Geometry: final body of the model. Coordinates: model frame, mm. Face numbers are marked on the shaded views. A direction names the side the tool comes from. Round coordinates to 2 decimals unless told otherwise and drop trailing zeros. Order: outer loops, then holes, each group sorted by start corner. A loop starts at its lowest first (then second) coordinate and runs counter-clockwise, first axis right, second up. Notation, with made-up numbers: (36, -30.75) -> (90, -30.75) arc R28 ccw to (90, -7.75) -> close; hole circle Ø1 at (37.25, 70). An arc over 180 degrees is marked (long way). Put each result on its own line as item: value.
```python
from build123d import *

# Parameters (mm, degrees)
SKETCH1_W                 = 44
SKETCH1_H                 = 57
BOSS_EXTRUDE1_DEPTH       = 2
BOSS_EXTRUDE2_DEPTH       = 3.5
BOSS_EXTRUDE2_DEPTH_BACK  = 2
SKETCH17_W                = 47.024890074
SKETCH17_H                = 2
BOSS_EXTRUDE7_DEPTH       = 38
SKETCH8_W                 = 31.89
SKETCH8_H                 = 7.76
BOSS_EXTRUDE5_DEPTH       = 9.38
SKETCH9_R                 = 2.4
CUT_EXTRUDE1_DEPTH        = 9.38
SKETCH10_R                = 3.1
CUT_EXTRUDE2_DEPTH        = 0.8
SKETCH11_R                = 3.1
CUT_EXTRUDE3_DEPTH        = 0.8
SKETCH14_R                = 2.4
CUT_EXTRUDE5_DEPTH        = 77.6
SKETCH15_R                = 3.1
CUT_EXTRUDE6_DEPTH        = 0.8
SKETCH16_R                = 3.1
CUT_EXTRUDE7_DEPTH        = 0.8
FILLET1_R                 = 1.3
FILLET2_R                 = 1.3
FILLET3_R                 = 1.3
FILLET4_R                 = 1.3
FILLET5_R                 = 1.3
FILLET7_R                 = 4
FILLET8_R                 = 4
FILLET9_R                 = 4
FILLET10_R                = 4
SKETCH19_W                = 3
SKETCH19_H                = 47
BOSS_EXTRUDE9_DEPTH       = 3.5
SKETCH20_W                = 25
SKETCH20_H                = 40
CUT_EXTRUDE8_DEPTH        = 10.38
SKETCH21_W                = 35
SKETCH21_H                = 50
CUT_EXTRUDE9_DEPTH        = 3.5
BOSS_EXTRUDE10_DEPTH      = 2.5
BOSS_EXTRUDE10_DEPTH_BACK = 2
FILLET11_R                = 2.5
FILLET12_R                = 2.5


with BuildPart() as part:
    # Sketch1 → Boss-Extrude1 (new body)
    with BuildSketch(Plane(origin=(0, 0, 0), x_dir=(1, 0, 0), z_dir=(0, 1, 0))):
        with Locations((22, 28.5)):
            Rectangle(SKETCH1_W, SKETCH1_H)
    extrude(amount=BOSS_EXTRUDE1_DEPTH)

    # Sketch2 → Boss-Extrude2 (add, two sides)
    with BuildSketch(Plane(origin=(0, 2, 0), x_dir=(1, 0, 0), z_dir=(0, 1, 0))) as boss_extrude2_sk:
        Polygon((0, 0), (0, 5), (-3, 5), (-3, 0), (-3, -3), (5, -3), (5, 0), align=None)
        Polygon((47, 0), (47, -3), (39, -3), (39, 0), (44, 0), (44, 5), (47, 5), align=None)
        Polygon((47, 57), (47, 52), (44, 52), (44, 57), (39, 57), (39, 60), (47, 60), align=None)
        Polygon((-3, 57), (-3, 60), (5, 60), (5, 57), (0, 57), (0, 52), (-3, 52), align=None)
    extrude(amount=BOSS_EXTRUDE2_DEPTH)
    extrude(boss_extrude2_sk.sketch, amount=-BOSS_EXTRUDE2_DEPTH_BACK)

    # Sketch17 → Boss-Extrude7 (add)
    with BuildSketch(Plane.ZY):
        with Locations((-28.487554963, 1)):
            Rectangle(SKETCH17_W, SKETCH17_H)
    extrude(amount=BOSS_EXTRUDE7_DEPTH)

    # Sketch8 → Boss-Extrude5 (add)
    with BuildSketch(Plane(origin=(0, 2, 0), x_dir=(1, 0, 0), z_dir=(0, 1, 0))):
        with Locations((22.150732417, 60.88)):
            Rectangle(SKETCH8_W, SKETCH8_H)
        with Locations((22.150732417, -3.88)):
            Rectangle(SKETCH8_W, SKETCH8_H)
    extrude(amount=-BOSS_EXTRUDE5_DEPTH)

    # Sketch9 → Cut-Extrude1 (cut)
    with BuildSketch(Plane(origin=(0, 0, -64.76), x_dir=(-1, 0, 0), z_dir=(0, 0, -1))):
        with Locations((-33.633843379, -3.383703118)):
            Circle(SKETCH9_R)
        with Locations((-25.663843379, -3.383703118)):
            Circle(SKETCH9_R)
        with Locations((-17.693843379, -3.383703118)):
            Circle(SKETCH9_R)
        with Locations((-9.723843379, -3.383703118)):
            Circle(SKETCH9_R)
    extrude(amount=-CUT_EXTRUDE1_DEPTH, mode=Mode.SUBTRACT)

    # Sketch10 → Cut-Extrude2 (cut)
    with BuildSketch(Plane(origin=(0, 0, -64.76), x_dir=(-1, 0, 0), z_dir=(0, 0, -1))):
        with Locations((-33.633843379, -3.383703118)):
            Circle(SKETCH10_R)
        with Locations((-25.663843379, -3.383703118)):
            Circle(SKETCH10_R)
        with Locations((-17.693843379, -3.383703118)):
            Circle(SKETCH10_R)
        with Locations((-9.723843379, -3.383703118)):
            Circle(SKETCH10_R)
    extrude(amount=-CUT_EXTRUDE2_DEPTH, mode=Mode.SUBTRACT)

    # Sketch11 → Cut-Extrude3 (cut)
    with BuildSketch(Plane.XY.offset(-57)):
        with Locations((33.633843379, -3.383703118)):
            Circle(SKETCH11_R)
        with Locations((25.633843379, -3.383703118)):
            Circle(SKETCH11_R)
        with Locations((17.633843379, -3.383703118)):
            Circle(SKETCH11_R)
        with Locations((9.633843379, -3.383703118)):
            Circle(SKETCH11_R)
    extrude(amount=-CUT_EXTRUDE3_DEPTH, mode=Mode.SUBTRACT)

    # Sketch14 → Cut-Extrude5 (cut)
    with BuildSketch(Plane.XY.offset(7.76)):
        with Locations((9.723843379, -3.383703118)):
            Circle(SKETCH14_R)
        with Locations((17.693843379, -3.383703118)):
            Circle(SKETCH14_R)
        with Locations((25.663843379, -3.383703118)):
            Circle(SKETCH14_R)
        with Locations((33.633843379, -3.383703118)):
            Circle(SKETCH14_R)
    extrude(amount=-CUT_EXTRUDE5_DEPTH, mode=Mode.SUBTRACT)

    # Sketch15 → Cut-Extrude6 (cut)
    with BuildSketch(Plane.XY.offset(7.76)):
        with Locations((9.723843379, -3.383703118)):
            Circle(SKETCH15_R)
        with Locations((17.693843379, -3.383703118)):
            Circle(SKETCH15_R)
        with Locations((25.663843379, -3.383703118)):
            Circle(SKETCH15_R)
        with Locations((33.633843379, -3.383703118)):
            Circle(SKETCH15_R)
    extrude(amount=-CUT_EXTRUDE6_DEPTH, mode=Mode.SUBTRACT)

    # Sketch16 → Cut-Extrude7 (cut)
    with BuildSketch(Plane(origin=(0, 0, 0), x_dir=(-1, 0, 0), z_dir=(0, 0, -1))):
        with Locations((-9.723843379, -3.383703118)):
            Circle(SKETCH16_R)
        with Locations((-17.693843379, -3.383703118)):
            Circle(SKETCH16_R)
        with Locations((-25.663843379, -3.383703118)):
            Circle(SKETCH16_R)
        with Locations((-33.633843379, -3.383703118)):
            Circle(SKETCH16_R)
    extrude(amount=-CUT_EXTRUDE7_DEPTH, mode=Mode.SUBTRACT)

    # Fillet1
    fillet1_edges = [part.edges().sort_by_distance(p)[0] for p in [
        (47, 5.5, -56),
        (43, 5.5, -60),
    ]]
    fillet(fillet1_edges, radius=FILLET1_R)

    # Fillet2
    fillet2_edges = [part.edges().sort_by_distance(p)[0] for p in [
        (47, 5.5, -1),
        (43, 5.5, 3),
    ]]
    fillet(fillet2_edges, radius=FILLET2_R)

    # Fillet3
    fillet3_edges = [part.edges().sort_by_distance(p)[0] for p in [
        (-3, 5.5, -56),
        (1, 5.5, -60),
    ]]
    fillet(fillet3_edges, radius=FILLET3_R)

    # Fillet4
    fillet4_edges = [part.edges().sort_by_distance(p)[0] for p in [
        (-3, 5.5, -1),
        (1, 5.5, 3),
    ]]
    fillet(fillet4_edges, radius=FILLET4_R)

    # Fillet5
    fillet5_edges = [part.edges().sort_by_distance(p)[0] for p in [
        (22.150732417, 2, -64.76),
    ]]
    fillet(fillet5_edges, radius=FILLET5_R)

    # Fillet7
    fillet7_edges = [part.edges().sort_by_distance(p)[0] for p in [
        (6.205732417, -7.38, -60.88),
    ]]
    fillet(fillet7_edges, radius=FILLET7_R)

    # Fillet8
    fillet8_edges = [part.edges().sort_by_distance(p)[0] for p in [
        (38.095732417, -7.38, -60.88),
    ]]
    fillet(fillet8_edges, radius=FILLET8_R)

    # Fillet9
    fillet9_edges = [part.edges().sort_by_distance(p)[0] for p in [
        (38.095732417, -7.38, 3.88),
    ]]
    fillet(fillet9_edges, radius=FILLET9_R)

    # Fillet10
    fillet10_edges = [part.edges().sort_by_distance(p)[0] for p in [
        (6.205732417, -7.38, 3.88),
    ]]
    fillet(fillet10_edges, radius=FILLET10_R)

    # Sketch19 → Boss-Extrude9 (add)
    with BuildSketch(Plane(origin=(0, 2, 0), x_dir=(1, 0, 0), z_dir=(0, 1, 0))):
        with Locations((-1.5, 28.5)):
            Rectangle(SKETCH19_W, SKETCH19_H)
    extrude(amount=BOSS_EXTRUDE9_DEPTH)

    # Sketch20 → Cut-Extrude8 (cut, through all)
    with BuildSketch(Plane(origin=(0, 2, 0), x_dir=(1, 0, 0), z_dir=(0, 1, 0))):
        with Locations((-20.5, 28.5)):
            Rectangle(SKETCH20_W, SKETCH20_H)
    extrude(amount=-CUT_EXTRUDE8_DEPTH, mode=Mode.SUBTRACT)

    # Sketch21 → Cut-Extrude9 (cut)
    with BuildSketch(Plane(origin=(0, 2, 0), x_dir=(1, 0, 0), z_dir=(0, 1, 0))):
        with Locations((22, 28.25)):
            Rectangle(SKETCH21_W, SKETCH21_H)
    extrude(amount=-CUT_EXTRUDE9_DEPTH, mode=Mode.SUBTRACT)

    # Sketch22 → Boss-Extrude10 (add, two sides)
    with BuildSketch(Plane(origin=(0, 2, 0), x_dir=(1, 0, 0), z_dir=(0, 1, 0))) as boss_extrude10_sk:
        Polygon((-38, 52), (-32.9998846, 52), (-32.9998846, 55.005068645), (-38, 55.005068645), (-40.988316888, 55.005068645), (-40.988316888, 46.981993776), (-38, 46.981993776), align=None)
        Polygon((-32.9998846, 4.975109926), (-32.9998846, 1.970041281), (-38, 1.970041281), (-40.988316888, 1.970041281), (-40.988316888, 9.99311615), (-38, 9.99311615), (-38, 4.975109926), align=None)
    extrude(amount=BOSS_EXTRUDE10_DEPTH)
    extrude(boss_extrude10_sk.sketch, amount=-BOSS_EXTRUDE10_DEPTH_BACK)

    # Fillet11
    fillet11_edges = [part.edges().sort_by_distance(p)[0] for p in [
        (-36.994100744, 4.5, -55.005068645),
        (-40.988316888, 4.5, -50.99353121),
    ]]
    fillet(fillet11_edges, radius=FILLET11_R)

    # Fillet12
    fillet12_edges = [part.edges().sort_by_distance(p)[0] for p in [
        (-40.988316888, 4.5, -5.981578716),
        (-36.994100744, 4.5, -1.970041281),
    ]]
    fillet(fillet12_edges, radius=FILLET12_R)


solid = part.part
```
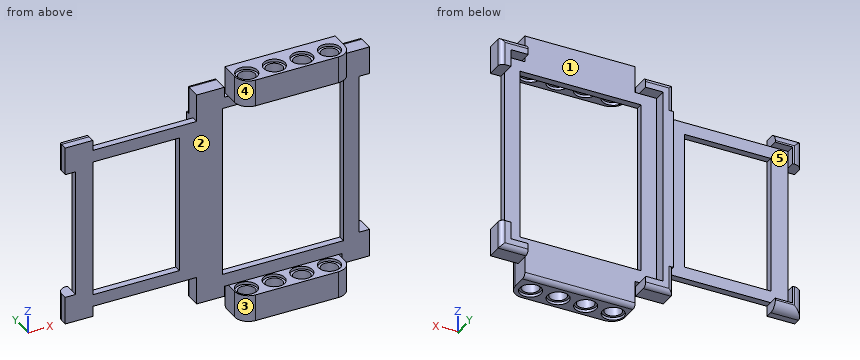
1. Material intervals for probe 1 along X at (y, z) = (-3.5, 3); probe 2 along Z at (x, y) = (4, 3.25); probe 3 along Z at (x, y) = (35, -5.5), sorted ascending.
Ans:
probe 1: 6.21 to 7.33, 12.12 to 15.3, 20.09 to 23.27, 28.06 to 31.24, 36.03 to 38.09
probe 2: -60 to -57, 0 to 3
probe 3: -63.96 to -57.8, 0.8 to 6.96
2. Contact query for flat-ended pins moving along their axis: P1, Ø4, axis at x = -14.5, z = -51, coming from the +Y side; P2, Ø2, axis at y = 1, z = -31, coming from the -X side; P3, Ø0.7, axis at x = 38.5, y = 1, coming from the +Z side; P4, Ø6, axis at y = -4, z = -33.5, coming from the -X side. Output: stop coordinate, or through.
Ans:
P1: y = 2
P2: x = -38
P3: z = 0
P4: through
3. Cut plane B-B on x = -17. Return loops of the section in (y, z).
Ans:
outline: (0, -52) -> (2, -52) -> (2, -48.5) -> (0, -48.5) -> close; (0, -8.5) -> (2, -8.5) -> (2, -4.98) -> (0, -4.98) -> close
4. Cut plane A-A on z = -35.5. Return loops of the section in (x, y), and give its area (3 significant figures).
Ans:
outline: (-38, 0) -> (-33, 0) -> (-33, 2) -> (-38, 2) -> close; (-8, 0) -> (4.5, 0) -> (4.5, 2) -> (0, 2) -> (0, 5.5) -> (-3, 5.5) -> (-3, 2) -> (-8, 2) -> close; (39.5, 0) -> (44, 0) -> (44, 2) -> (39.5, 2) -> close
area: 54.5 mm²
5. Cut plane D-D on x = 33. State how many separate pieces and enclosed holes the cut face has, and give its area (3 significant figures).
Ans:
separate pieces: 4
enclosed holes: 0
area: 82.8 mm²
6. Cut plane C-C on z = -56. Return loops of the section in (x, y), and give its area (3 significant figures).
Ans:
outline: (-3, 0) -> (47, 0) -> (47, 4.2) arc R1.3 ccw to (45.7, 5.5) -> (44, 5.5) -> (44, 2) -> (0, 2) -> (0, 5.5) -> (-1.7, 5.5) arc R1.3 ccw to (-3, 4.2) -> close
area: 120 mm²
7. Draft query along X for the marked faces 1, 2 and 3. Return one class per face: +X half, -X half, draft (parallel to the pull), parting line (faces both ways), or undercut.
Ans:
face 1: undercut
face 2: draft
face 3: -X half
8. Set-up query: the marked faces 4 and 5. Return all of +Z, -Z, +X, -X, +Y, -Y with unobstructed straight access to the full face (end or side cutting, diameter ignored); none if empty.
Ans:
face 4: +Z, -Z, -X, -Y
face 5: +Y
